Can you work these out from the model? Positions are in its coordinate system, mm. A direction names the side the tool comes from. Give positions to 0.01 mm unless a question says otherwise; leave off trailing zeros. Order: outer loops, then holes, each group sorted by start corner. A loop starts at its lowest first (then second) coordinate and runs counter-clockwise, first axis right, second up.
Item 1: If I drill on line 1 along Y through (x, z) = (171, 308); line 2 along X through (y, z) = (24, 179); line 3 along X through (y, z) = (-9, 230), over which ranges is the centre line in solid material (lowest first)?
Item 2: I want a section at C-C, the plane x = 91.5. Write out the boundary of the cut face in (y, z), then the cut area to 3 significant figures.
Item 3: I'm going to push a flat-ended pin straight in: pin 1 Ø12 at (x, z) = (99, 68.5) entering from +Y. Where does the tip first touch, or does it pass through?
Item 4: I want a section at A-A, the plane y = 26. Write out the boundary of the cut face in (x, z).
Item 5: Which directions (+Z, -Z, +X, -X, +Y, -Y) give clear straight access to the entire face, cutting with the end or side of a thin tool? Please do faces 1 (the flat face through (150, 25, 145)), 2 (the flat face through (200, -1, -10)), 3 (the flat face through (101, -12.5, 145)).
Item 6: I want a section at B-B, the plane z = 302.5. Write out the boundary of the cut face in (x, y).
Item 7: If we mould it in two halves opening along Y, with no side actions, what happens to faces 4 (the flat face through (37, 12.5, 145)), 5 (the flat face through (50, 25, 145)), 6 (the flat face through (99, -37.5, -10))? For each: +Y half, -Y half, draft (parallel to the pull), parting line (faces both ways), or undercut.
```python
from build123d import *

# Parameters (mm, degrees)
F0_W     = 75
F0_H     = 610
F1_DEPTH = 200
F2_W     = 25
F2_H     = 25
F3_DEPTH = 525
F4_W     = 200
F4_H     = 75
F5_DEPTH = 220
F7_DEPTH = 215


with BuildPart() as f1:
    # F0 (on Right) → F1 (new body)
    with BuildSketch(Plane.YZ):
        Rectangle(F0_W, F0_H)
    extrude(amount=F1_DEPTH)

    # F2 (on face) → F3 (cut)
    with BuildSketch(Plane.XY.offset(305)):
        Polygon((150, 37.5), (50, 37.5), (50, 12.5), (50, -12.5), (150, -12.5), (150, 12.5), align=None)
        with Locations((37.5, 0)):
            Rectangle(F2_W, F2_H)
        with Locations((162.5, 0)):
            Rectangle(F2_W, F2_H)
    extrude(amount=-F3_DEPTH, mode=Mode.SUBTRACT)

    # F4 (on face) → F5 (join)
    with BuildSketch(Plane(origin=(0, 0, -305), x_dir=(1, 0, 0), z_dir=(0, 0, -1))):
        with Locations((100, 0)):
            Rectangle(F4_W, F4_H)
    extrude(amount=F5_DEPTH)

    # F6 (on face) → F7 (join)
    with BuildSketch(Plane.XY.offset(305)):
        Polygon((25, -12.5), (25, 12.5), (50, 12.5), (50, 37.5), (0, 37.5), (0, -37.5), (200, -37.5), (200, 37.5), (150, 37.5), (150, 12.5), (175, 12.5), (175, -12.5), align=None)
    extrude(amount=F7_DEPTH)


solid = f1.part
```
Results list:
1. line 1: y = -37.5 to -12.5, 12.5 to 37.5
1. line 2: x = 0 to 50, 150 to 200
1. line 3: x = 0 to 25, 175 to 200
2. outline: (-37.5, -525) - (37.5, -525) - (37.5, -220) - (-12.5, -220) - (-12.5, 520) - (-37.5, 520) - close
2. area: 41,400 mm2
3. pin 1: stops at y = -12.5
4. outline: (0, -525) - (200, -525) - (200, 520) - (150, 520) - (150, -220) - (50, -220) - (50, 520) - (0, 520) - close
5. face 1: +Z, +Y
5. face 2: +Z, -Z, +X, +Y, -Y
5. face 3: +Z
6. outline: (0, -37.5) - (200, -37.5) - (200, 37.5) - (150, 37.5) - (150, 12.5) - (175, 12.5) - (175, -12.5) - (25, -12.5) - (25, 12.5) - (50, 12.5) - (50, 37.5) - (0, 37.5) - close
7. face 4: undercut
7. face 5: draft
7. face 6: -Y half
